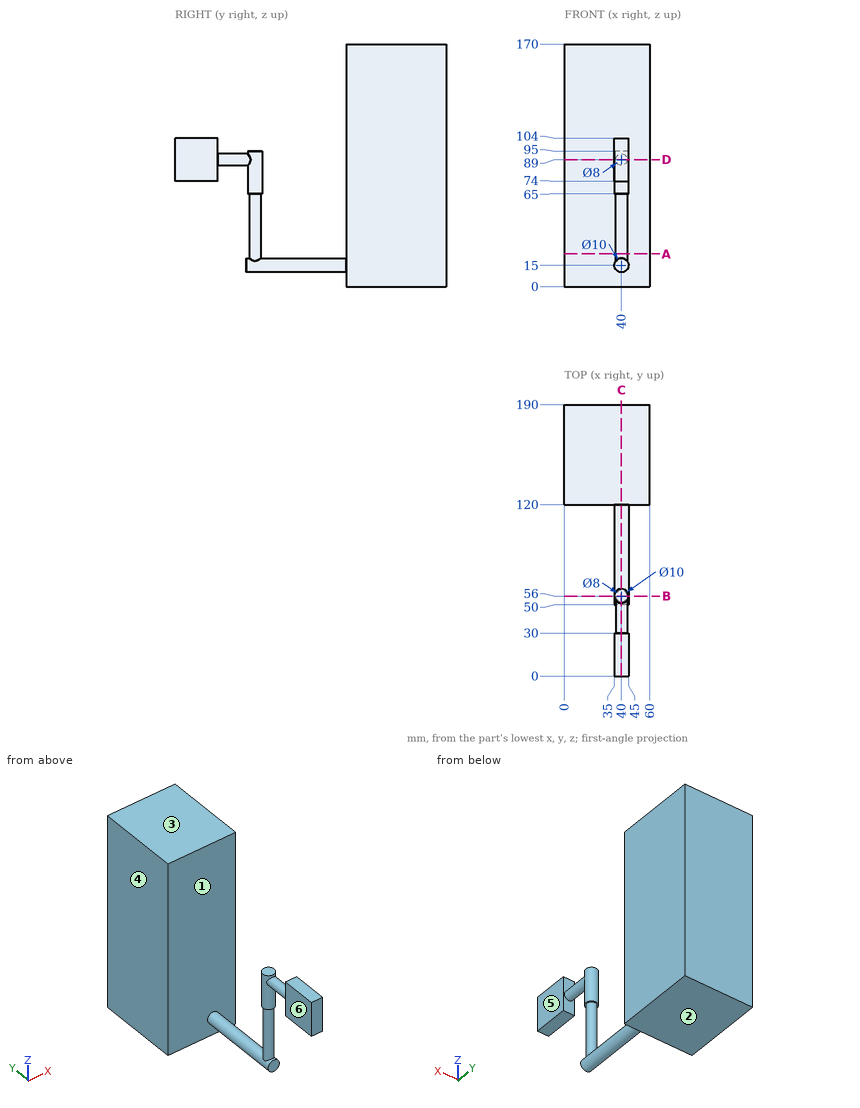
Input: dimensioned drawing with shaded views. Units: mm. Origin: part minimum x, y, z. A direction names the side the tool comes from. Round coordinates to 2 decimals unless told otherwise and drop trailing zeros. Loops run counter-clockwise (first coordinate to the right, second up) from the corner with the lowest first, then second, coordinate; pieces in that order, holes last.
1) Set-up query: the marked faces 4, 5 and 6. Return all of +Z, -Z, +X, -X, +Y, -Y with unobstructed straight access to the full face (end or side cutting, diameter ignored); none if empty.
Ans:
face 4: +Z, -Z, -X, +Y, -Y
face 5: +Z, -Z, +X, -Y
face 6: +Z, -Z, -X, -Y
2) Section query A-A on z = 23. Return the cut outline in (x, y), plus the area to 3 significant figures.
Ans:
outline: (0, 120) - (60, 120) - (60, 190) - (0, 190) - close; circle Ø8 at (40, 56)
area: 4,250 mm2
3) Section query D-D on z = 89. Return the cut outline in (x, y).
Ans:
outline: (0, 120) - (60, 120) - (60, 190) - (0, 190) - close; (35, 0) - (45, 0) - (45, 30) - (44, 30) - (44, 53) arc R5 ccw (long way) to (36, 53) - (36, 30) - (35, 30) - close
4) Section query C-C on x = 40. Return the cut outline in (y, z).
Ans:
outline: (0, 74) - (30, 74) - (30, 85) - (51, 85) - (51, 65) - (52, 65) - (52, 20) - (50, 20) - (50, 10) - (120, 10) - (120, 0) - (190, 0) - (190, 170) - (120, 170) - (120, 20) - (60, 20) - (60, 65) - (61, 65) - (61, 95) - (51, 95) - (51, 93) - (30, 93) - (30, 104) - (0, 104) - close
5) Material intervals for line 1 (Y direction, x = 39, z = 127); line 2 (Y direction, x = 41, z = 33); line 3 (X direction, y = 109.5, z = 11.5), sorted ascending.
Ans:
line 1: y = 120 to 190
line 2: y = 52.13 to 59.87, 120 to 190
line 3: x = 36.43 to 43.57
6) Section query B-B on y = 56. Return the cut outline in (x, z), plus the area to 3 significant figures.
Ans:
outline: (35, 65) - (36, 65) - (36, 18) arc R5 ccw (long way) to (44, 18) - (44, 65) - (45, 65) - (45, 95) - (35, 95) - close
area: 743 mm2
7) Pull-direction query (Z, two-part tool) for the marked faces 1, 2 and 3; classes: released by +Z, released by -Z, zero draft, split by the parting line, or undercut.
Ans:
face 1: zero draft
face 2: released by -Z
face 3: released by +Z
8) Pin query (flat end, axial travel): pin 1 (1 mm diameter, centred on x = 42.5, y = 102.5, fed in from +Z); pin 2 (8 mm diameter, centred on y = 158, z = 41.5, fed in from -X); pin 3 (24 mm diameter, centred on y = 10.5, z = 92.5, fed in from +X); pin 4 (8 mm diameter, centred on x = 37.5, z = 16.5, fed in from -Y). Return the tip coordinate at first contact, or that it passes through.
Ans:
pin 1: stops at z = 19.58
pin 2: stops at x = 0
pin 3: stops at x = 45
pin 4: stops at y = 50
